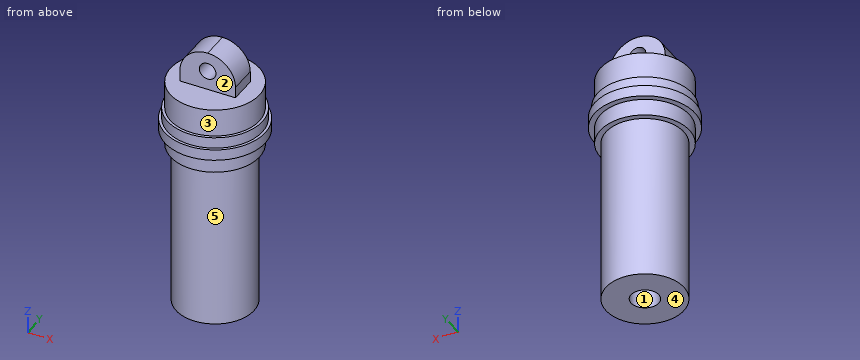
Autodesk Inventor part; units mm, degrees
ref_plane "YZ Plane" through (0, 0, 0) normal (1, 0, 0) x (0, 1, 0)
ref_plane "XZ Plane" through (0, 0, 0) normal (0, 1, 0) x (-1, 0, 0)
ref_plane "XY Plane" through (0, 0, 0) normal (0, 0, 1) x (1, 0, 0)
sketch "スケッチ1" plane through (0, 0, 0) normal (0, 0, 1) x (1, 0, 0)
  circle A0 centre (0, 0) radius 7
  circle A1 centre (0, 0) radius 2.5
  dimension "d0" = 14
  dimension "d1" = 5
extrude "押し出し1" add sketch "スケッチ1" along normal blind 30
sketch "スケッチ2" plane through (0, 0, 30) normal (0, 0, 1) x (1, 0, 0)
  circle A0 centre (0, 0) radius 8
  dimension "d4" = 16
extrude "押し出し2" add sketch "スケッチ2" along normal blind 3
sketch "スケッチ3" plane through (0, 0, 33) normal (0, 0, 1) x (1, 0, 0)
  circle A0 centre (0, 0) radius 9
  dimension "d7" = 18
extrude "押し出し3" add sketch "スケッチ3" along normal blind 2
sketch "スケッチ4" plane through (0, 0, 35) normal (0, 0, 1) x (1, 0, 0)
  circle A0 centre (0, 0) radius 8.5
  dimension "d10" = 17
extrude "押し出し4" add sketch "スケッチ4" along normal blind 2
sketch "スケッチ5" plane through (0, 0, 37) normal (0, 0, 1) x (1, 0, 0)
  circle A0 centre (0, 0) radius 8
  dimension "d13" = 16
extrude "押し出し5" add sketch "スケッチ5" along normal blind 5
sketch "スケッチ6" plane through (0, 0, 42) normal (0, 0, 1) x (1, 0, 0)
  line L0 (-5, -2.5) -> (5, -2.5)
  line L1 (5, -2.5) -> (5, 2.5)
  line L2 (5, 2.5) -> (-5, 2.5)
  line L3 (-5, 2.5) -> (-5, -2.5)
  line L4 (-5, -2.5) -> (5, 2.5) construction
  line L5 (5, -2.5) -> (-5, 2.5) construction
  point P0 (0, 0)
  dimension "d16" = 10
  dimension "d17" = 5
extrude "押し出し6" add sketch "スケッチ6" along normal blind 7
fillet "フィレット1" radius 5 1 edges at (-5, 0, 49)
fillet "フィレット2" radius 5 1 edges at (5, 0, 49)
sketch "スケッチ7" plane through (-5, -2.5, 42) normal (0, -1, 0) x (1, 0, 0)
  arc A0 (10, 2) -> (0, 2) centre (5, 2) ccw
  line L0 (0, 0) -> (0, 2)
  line L1 (10, 0) -> (0, 0)
  line L2 (10, 0) -> (10, 2)
  circle A1 centre (5, 3.5) radius 1.5
  point P0 (5, -42)
  dimension "d22" = 3
  dimension "d23" = 2
extrude "押し出し7" cut sketch "スケッチ7" against normal blind 8 contours A1
properties part number "タミヤダンパー"
Verification items for the finished model (mm, model axes). Face numbers are marked on the shaded views. A direction names the side the tool comes from. Round coordinates to 2 decimals unless told otherwise and drop trailing zeros. Order: outer loops, then holes, each group sorted by start corner. A loop starts at its lowest first (then second) coordinate and runs counter-clockwise, first axis right, second up.
1. Go/stop test with flat-tipped pins: P1, Ø10, axis at y = 1, z = 23.5, coming from the -X side; P2, Ø5, axis at x = 0, z = 45.5, coming from the -Y side; P3, Ø7.5, axis at x = 0, z = 45, coming from the +Y side. Record where each tip stops, or that it passes through.
Final values:
P1: stops at x = -7
P2: stops at y = -2.5
P3: stops at y = 8
2. Access from +Z, -Z, +X, -X, +Y, -Y to the whole of each face (thin tool, end or side, straight path). Record for the marked faces 4 and 5.
Final values:
face 4: -Z, +X, -X, +Y, -Y
face 5: -Z
3. Section check D-D on y = -4. Record the cut outline in (x, z), then the cut area to 3 significant figures.
Final values:
outline: (-8.06, 33) - (-6.93, 33) - (-6.93, 30) - (-5.74, 30) - (-5.74, 0) - (5.74, 0) - (5.74, 30) - (6.93, 30) - (6.93, 33) - (8.06, 33) - (8.06, 35) - (7.5, 35) - (7.5, 37) - (6.93, 37) - (6.93, 42) - (-6.93, 42) - (-6.93, 37) - (-7.5, 37) - (-7.5, 35) - (-8.06, 35) - close
area: 518 mm2
4. Release check for a two-part mould opening along X. For the marked faces 1, 2 and 3 record: +X half, -X half, draft (parallel to the pull), parting line (faces both ways), or undercut.
Final values:
face 1: undercut
face 2: draft
face 3: parting line
5. Section check C-C on x = 2. Record the cut outline in (y, z), then the cut area to 3 significant figures.
Final values:
outline: (-8.77, 33) - (-7.75, 33) - (-7.75, 30) - (-6.71, 30) - (-6.71, 0) - (-1.5, 0) - (-1.5, 30) - (1.5, 30) - (1.5, 0) - (6.71, 0) - (6.71, 30) - (7.75, 30) - (7.75, 33) - (8.77, 33) - (8.77, 35) - (8.26, 35) - (8.26, 37) - (7.75, 37) - (7.75, 42) - (2.5, 42) - (2.5, 48.58) - (-2.5, 48.58) - (-2.5, 42) - (-7.75, 42) - (-7.75, 37) - (-8.26, 37) - (-8.26, 35) - (-8.77, 35) - close
area: 537 mm2
6. Thickness scan on L1, parallel to Z at x = 0, y = 0.3; L2, parallel to Y at x = 0, z = 18.5; L3, parallel to Z at x = -7, y = -1. Record the ranges inside material, lowest first.
Final values:
L1: z = 30 to 44, 47 to 49
L2: y = -7 to -2.5, 2.5 to 7
L3: z = 30 to 42
7. Section check B-B on z = 45.5. Record the cut outline in (x, y).
Final values:
outline: (-4.77, -2.5) - (-1.5, -2.5) - (-1.5, 2.5) - (-4.77, 2.5) - close; (1.5, -2.5) - (4.77, -2.5) - (4.77, 2.5) - (1.5, 2.5) - close
